from build123d import *

# Parameters (mm, degrees)
F0_W           = 50
F0_H           = 82
F0_W_2         = 35
F0_H_2         = 70
F1_DEPTH       = 3.81
F3_D           = 2
F3_DEPTH       = 50.8
F3_CSINK_D     = 3.5
F3_CSINK_ANGLE = 90


with BuildPart() as f1:
    # F0 (on Right) → F1 (new body)
    with BuildSketch(Plane.YZ):
        with Locations((-0.991207, 6.902988)):
            Rectangle(F0_W, F0_H)
        with Locations((-1.261404, 7.01166)):
            Rectangle(F0_W_2, F0_H_2, mode=Mode.SUBTRACT)
    extrude(amount=F1_DEPTH)

    # F3
    with Locations(Plane.YZ.offset(3.81)):
        with Locations((-23.991207, 45.902988), (22.008793, 45.902988), (22.008793, -32.097012), (-23.991207, -32.097012)):
            CounterSinkHole(F3_D / 2, F3_CSINK_D / 2, depth=F3_DEPTH, counter_sink_angle=F3_CSINK_ANGLE)


solid = f1.part
The listing builds one solid part. Answer for the finished solid, in the listing's coordinates (mm). A direction names the side the tool comes from. Give positions to 0.01 mm unless a question says otherwise; leave off trailing zeros. Loops run counter-clockwise (first coordinate to the right, second up) from the corner with the lowest first, then second, coordinate; pieces in that order, holes last. Notation, with made-up numbers: (-34.5, -18.5) - (-25.5, -18.5) arc R21 ccw to (-25.5, 5.5) - close; hole circle Ø1 at (77.5, -2.75). An arc over 180 degrees is marked (long way). Write each question's results on one line, items separated by ' | '.
1. Consider probe 1 along Y at (x, z) = (0.8, 4); probe 2 along Z at (x, y) = (2.3, -1). Determine where each line is inside the solid, lowest interval first. Write a range as from..to.
Resolved:
probe 1: y = -25.99..-18.76, 16.24..24.01 | probe 2: z = -34.1..-27.99, 42.01..47.9
2. Find section C-C, the plane x = 1.2. Write down the section's boundary in (y, z), then the cut area to 3 significant figures.
Resolved:
outline: (-25.99, -34.1) - (24.01, -34.1) - (24.01, 47.9) - (-25.99, 47.9) - close; hole circle Ø2 at (-23.99, -32.1); hole circle Ø2 at (-23.99, 45.9); hole (-18.76, -27.99) - (16.24, -27.99) - (16.24, 42.01) - (-18.76, 42.01) - close; hole circle Ø2 at (22.01, -32.1); hole circle Ø2 at (22.01, 45.9) | area: 1,640 mm^2
3. For a pull along Y with two mould halves and no side action, classify faces 1 (the face through (0, -24, 7)), 2 (the face through (1.509, 22.226, 44.927)), 3 (the face through (2, -25.991, 6)) as +Y half, -Y half, draft (parallel to the pull), parting line (faces both ways), or undercut.
Resolved:
face 1: draft | face 2: undercut | face 3: -Y half
4. Find section B-B, the plane y = -3. Write down the section's boundary in (x, z), then the cut area to 3 significant figures.
Resolved:
outline: (0, -34.1) - (3.81, -34.1) - (3.81, -27.99) - (0, -27.99) - close; (0, 42.01) - (3.81, 42.01) - (3.81, 47.9) - (0, 47.9) - close | area: 45.7 mm^2
5. Which of the six approach directions +Z, -Z, +X, -X, +Y, -Y give full straight-line access (tool end or side, diameter ignored) to faces 4 (the face through (2, -1, 47.903)), 5 (the face through (2, -2, -27.988))?
Resolved:
face 4: +Z, +X, -X, +Y, -Y | face 5: +X, -X
6. Flat-ended cylindrical pins translate along their axes: P1, Ø1.8, axis at y = 22.01, z = 45.9, coming from the -X side; P2, Ø3, axis at y = 22.01, z = -32.1, coming from the +X side. Find the tip coordinate at first contact, or state that the pin passes through.
Resolved:
P1: passes through | P2: stops at x = 3.56
7. Find section A-A, the plane z = 6. Write down the section's boundary in (x, y).
Resolved:
outline: (0, -25.99) - (3.81, -25.99) - (3.81, -18.76) - (0, -18.76) - close; (0, 16.24) - (3.81, 16.24) - (3.81, 24.01) - (0, 24.01) - close
